from build123d import *

# Parameters (mm, degrees)
SKETCH1_R               = 55
BOSS_EXTRUDE1_DEPTH     = 15.5
SKETCH2_R               = 44.25
BOSS_EXTRUDE2_DEPTH     = 15
SKETCH3_R               = 44
CUT_EXTRUDE1_DEPTH      = 7
CUT_EXTRUDE2_DEPTH      = 82.254230659
CUT_EXTRUDE2_DEPTH_BACK = 82.254230659
SKETCH4_R               = 37.5


with BuildPart() as part:
    # Sketch1 → Boss-Extrude1 (new body)
    with BuildSketch(Plane.XY):
        Circle(SKETCH1_R)
    extrude(amount=BOSS_EXTRUDE1_DEPTH)

    # Sketch2 → Boss-Extrude2 (add)
    with BuildSketch(Plane.XY.offset(15.5)):
        Circle(SKETCH2_R)
    extrude(amount=BOSS_EXTRUDE2_DEPTH)

    # Sketch3 → Cut-Extrude1 (cut)
    with BuildSketch(Plane(origin=(0, 0, 0), x_dir=(-1, 0, 0), z_dir=(0, 0, -1))):
        Circle(SKETCH3_R)
    extrude(amount=-CUT_EXTRUDE1_DEPTH, mode=Mode.SUBTRACT)

    # Sketch4 → Cut-Extrude2 (cut, two sides: drawn at the far end of the back side and taken through both)
    with BuildSketch(Plane(origin=(0, 0, 7), x_dir=(-1, 0, 0), z_dir=(0, 0, -1)).offset(-CUT_EXTRUDE2_DEPTH_BACK)):
        Circle(SKETCH4_R)
    extrude(amount=CUT_EXTRUDE2_DEPTH + CUT_EXTRUDE2_DEPTH_BACK, mode=Mode.SUBTRACT)


solid = part.part
Build history of the part. All positions in model axes, mm. A direction names the side the tool comes from. Round coordinates to 2 decimals unless told otherwise and drop trailing zeros. Write each loop counter-clockwise with the first axis right and the second up, starting at its lowest first coordinate (ties: lowest second). Pieces come first, ordered by that corner, then holes. Notation, with made-up numbers: M 44,-26 L 70,-26 A18 ccw 70,-3 Z; hole C 30.5,-40 d8. An arc over 180 degrees is marked long. Answer as a JSON object with one key per item and string values. Group by question number.
(1) Cut at D-D (y = -40.5). Give the cut face in (x, z), and give its area (3 significant figures).
(2) Mould opens along Y. For faces 1 (the cylindrical face through (-11.923, -53.692, 7.642)), 2 (the flat face through (-37, 25, 15.5)), 3 (the cylindrical face through (4.88, 37.18, 18.91)) say: pulls with the +Y half, pulls with the -Y half, needs draft (parallel to the pull), parting line crosses it, or undercut.
(3) Flat gauge pins, fed straight in: pin 1 (4 mm diameter, centred on y = -11.5, z = 14, fed in from +X); pin 2 (4 mm diameter, centred on y = 4.5, z = 16.5, fed in from -X); pin 3 (6 mm diameter, centred on x = -13.5, z = 20.5, fed in from -Y). Where does each tip first touch, or does it go through?
(4) Drill centre lines: L1, parallel to Y at x = 0, z = 13.75; L2, parallel to Y at x = 0, z = 4; L3, parallel to Z at x = 47.5, y = -13. Where is each one in solid material? Low to high.
(5) Which spindle directions (+Z, -Z, +X, -X, +Y, -Y) get a long thin tool onto all of the face, cutting with end or side? Do faces 4 (the cylindrical face through (-9.59, -43.2, 22.9)), 5 (the flat face through (-32, 20, 7)), 6 (the flat face through (-36.3, 10, 30.5)). Say none if no direction does.
(6) Cut at C-C (z = 4). Give the cut face in (x, y), and give its area (3 significant figures).
(7) Cut at A-A (y = 0). Give the cut face in (x, z).
Responses:
{
 "1": {"outline": "M -37.21,0 L -17.2,0 L -17.2,7 L 17.2,7 L 17.2,0 L 37.21,0 L 37.21,15.5 L 17.83,15.5 L 17.83,30.5 L -17.83,30.5 L -17.83,15.5 L -37.21,15.5 Z", "area": "1,450 mm2"},
 "2": {"face 1": "parting line crosses it", "face 2": "needs draft", "face 3": "undercut"},
 "3": {"pin 1": "stops at x = 54.17", "pin 2": "stops at x = -54.93", "pin 3": "stops at y = -42.99"},
 "4": {"L1": "y = -55 to -37.5, 37.5 to 55", "L2": "y = -55 to -44, 44 to 55", "L3": "z = 0 to 15.5"},
 "5": {"face 4": "+Z", "face 5": "-Z", "face 6": "+Z, +X, -X, +Y, -Y"},
 "6": {"outline": "C 0,0 d110; hole C 0,0 d88", "area": "3,420 mm2"},
 "7": {"outline": "M -55,0 L -44,0 L -44,7 L -37.5,7 L -37.5,30.5 L -44.25,30.5 L -44.25,15.5 L -55,15.5 Z; M 37.5,7 L 44,7 L 44,0 L 55,0 L 55,15.5 L 44.25,15.5 L 44.25,30.5 L 37.5,30.5 Z"}
}
